Work out the finished part from the listing and answer in its coordinate system (mm). A direction names the side the tool comes from. Round coordinates to 2 decimals unless told otherwise and drop trailing zeros. Write each loop counter-clockwise with the first axis right and the second up, starting at its lowest first coordinate (ties: lowest second). Pieces come first, ordered by that corner, then holes. Notation, with made-up numbers: (76, 43.25) - (98, 43.25) arc R23 ccw to (98, 55.25) - close; hole circle Ø3 at (0, 36.25). An arc over 180 degrees is marked (long way). Answer as a JSON object with one key per item and string values.
```python
from build123d import *

# Parameters (mm, degrees)
SKETCH1_W           = 76.2
SKETCH1_H           = 88.9
SKETCH1_W_2         = 63.5
SKETCH1_H_2         = 76.2
BOSS_EXTRUDE1_DEPTH = 3.175
SKETCH2_W           = 5.334
SKETCH2_H           = 3.429
SKETCH2_W_2         = 3.429
SKETCH2_H_2         = 5.08
CUT_EXTRUDE1_DEPTH  = 59.630138368


with BuildPart() as part:
    # Sketch1 → Boss-Extrude1 (new body)
    with BuildSketch(Plane(origin=(0, 0, 0), x_dir=(1, 0, 0), z_dir=(0, 1, 0))):
        Rectangle(SKETCH1_W, SKETCH1_H)
        Rectangle(SKETCH1_W_2, SKETCH1_H_2, mode=Mode.SUBTRACT)
    extrude(amount=BOSS_EXTRUDE1_DEPTH)

    # Sketch2 → Cut-Extrude1 (cut, through all)
    with BuildSketch(Plane(origin=(0, 0, 0), x_dir=(1, 0, 0), z_dir=(0, 1, 0))):
        with Locations((20.447, -42.7355)):
            Rectangle(SKETCH2_W, SKETCH2_H)
        with Locations((10.287, -42.7355)):
            Rectangle(SKETCH2_W, SKETCH2_H)
        with Locations((0.127, -42.7355)):
            Rectangle(SKETCH2_W, SKETCH2_H)
        with Locations((-10.033, -42.7355)):
            Rectangle(SKETCH2_W, SKETCH2_H)
        with Locations((-20.32, -42.7355)):
            Rectangle(SKETCH2_W, SKETCH2_H)
        with Locations((-36.3855, 35.56)):
            Rectangle(SKETCH2_W_2, SKETCH2_H_2)
        with Locations((-36.3855, 25.4)):
            Rectangle(SKETCH2_W_2, SKETCH2_H_2)
        with Locations((-36.3855, 15.24)):
            Rectangle(SKETCH2_W_2, SKETCH2_H_2)
        with Locations((-36.3855, 5.08)):
            Rectangle(SKETCH2_W_2, SKETCH2_H_2)
        with Locations((-36.3855, -5.08)):
            Rectangle(SKETCH2_W_2, SKETCH2_H_2)
        with Locations((-36.3855, -15.24)):
            Rectangle(SKETCH2_W_2, SKETCH2_H_2)
        with Locations((-36.3855, -25.4)):
            Rectangle(SKETCH2_W_2, SKETCH2_H_2)
        with Locations((-36.3855, -35.56)):
            Rectangle(SKETCH2_W_2, SKETCH2_H_2)
        with Locations((36.3855, -35.56)):
            Rectangle(SKETCH2_W_2, SKETCH2_H_2)
        with Locations((36.3855, -25.4)):
            Rectangle(SKETCH2_W_2, SKETCH2_H_2)
        with Locations((36.3855, -15.24)):
            Rectangle(SKETCH2_W_2, SKETCH2_H_2)
        with Locations((36.3855, -5.08)):
            Rectangle(SKETCH2_W_2, SKETCH2_H_2)
        with Locations((36.3855, 5.08)):
            Rectangle(SKETCH2_W_2, SKETCH2_H_2)
        with Locations((36.3855, 15.24)):
            Rectangle(SKETCH2_W_2, SKETCH2_H_2)
        with Locations((36.3855, 25.4)):
            Rectangle(SKETCH2_W_2, SKETCH2_H_2)
        with Locations((36.3855, 35.56)):
            Rectangle(SKETCH2_W_2, SKETCH2_H_2)
        with Locations((-20.32, 42.7355)):
            Rectangle(SKETCH2_W, SKETCH2_H)
        with Locations((-10.033, 42.7355)):
            Rectangle(SKETCH2_W, SKETCH2_H)
        with Locations((0.127, 42.7355)):
            Rectangle(SKETCH2_W, SKETCH2_H)
        with Locations((10.287, 42.7355)):
            Rectangle(SKETCH2_W, SKETCH2_H)
        with Locations((20.447, 42.7355)):
            Rectangle(SKETCH2_W, SKETCH2_H)
    extrude(amount=CUT_EXTRUDE1_DEPTH, mode=Mode.SUBTRACT)


solid = part.part
```
Item 1: A cutting plane is placed at B-B (z = -37). Write down the section's boundary in (x, y) (3 decimals), and give its area (3 significant figures).
Results found:
{"outline": "(-34.671, 0) - (-31.75, 0) - (-31.75, 3.175) - (-34.671, 3.175) - close; (31.75, 0) - (34.671, 0) - (34.671, 3.175) - (31.75, 3.175) - close", "area": "18.5 mm²"}
Item 2: Determine the mould class of faces 6 (the flat face through (-38.1, 2, 20)), 7 (the flat face through (-15, 2, -44.45)), 8 (the flat face through (-10, 2, -41.021)) for opening direction X: pulls with the +X half, pulls with the -X half, needs draft (parallel to the pull), parting line crosses it, or undercut.
Results found:
{"face 6": "pulls with the -X half", "face 7": "needs draft", "face 8": "undercut"}
Item 3: For faces 1 (the flat face through (36, 2, -7.62)), 2 (the flat face through (38.1, 2, 31)), 3 (the flat face through (-12.7, 2, 43)), 4 (the flat face through (-36, 2, 27.94)), 5 (the flat face through (-17.653, 2, -43)), determine the directions among +Z, -Z, +X, -X, +Y, -Y from which every point of the face is accessible in a straight line to the end or side of a thin tool.
Results found:
{"face 1": "+X, +Y, -Y", "face 2": "+Z, -Z, +X, +Y, -Y", "face 3": "+Z, +Y, -Y", "face 4": "-X, +Y, -Y", "face 5": "-Z, +Y, -Y"}
Item 4: This flat-tipped pin is pushed along its axis until it touches: P1, Ø1.5, axis at y = 2, z = 34.5, coming from the +X side. Where does it stop, or does it pass through?
Results found:
{"P1": "x = 34.67"}
Item 5: A cutting plane is placed at A-A (x = -29). Write down the section's boundary in (y, z) (3 decimals), and give its area (3 significant figures).
Results found:
{"outline": "(0, -44.45) - (3.175, -44.45) - (3.175, -38.1) - (0, -38.1) - close; (0, 38.1) - (3.175, 38.1) - (3.175, 44.45) - (0, 44.45) - close", "area": "40.3 mm²"}
Item 6: Consider line 1 along X through (y, z) = (1.15, 12.5); line 2 along Z through (x, y) = (24, 1.35); line 3 along X through (y, z) = (0.85, 4.5). Determine where each line is inside the solid, lowest interval first.
Results found:
{"line 1": "-38.1 to -31.75, 31.75 to 38.1", "line 2": "-44.45 to -38.1, 38.1 to 44.45", "line 3": "-34.67 to -31.75, 31.75 to 34.67"}
